from build123d import *

# Parameters (mm, degrees)
F0_W         = 26
F0_H         = 16
F0_W_2       = 20
F0_H_2       = 10
F1_DEPTH     = 20
F3_DEPTH     = 50
F4_SIZE      = 3
F5_T1_DEPTH  = 10
F5_T3_DEPTH  = 20
F5_T5_DEPTH  = 9.3860066631
F5_T7_DEPTH  = 9.3860066631
F5_T9_DEPTH  = 9.3860066631
F5_T11_DEPTH = 9.3860066631
F5_T13_DEPTH = 25.1433659759
F5_T15_DEPTH = 15.1433659759
F5_T21_DEPTH = 22.571682988
F5_T25_DEPTH = 12.571682988
F5_T32_DEPTH = 22.571682988
F5_T36_DEPTH = 12.571682988
F5_T43_DEPTH = 12.571682988
F5_T47_DEPTH = 22.571682988
F5_T54_DEPTH = 22.571682988
F5_T58_DEPTH = 12.571682988
F6_T1_DEPTH  = 9.3860066631
F6_T3_DEPTH  = 10
F6_T5_DEPTH  = 9.3860066631
F6_T7_DEPTH  = 25.1433659759
F6_T9_DEPTH  = 20
F6_T14_DEPTH = 9.3860066631
F6_T19_DEPTH = 9.3860066631
F6_T25_DEPTH = 22.571682988
F6_T30_DEPTH = 12.571682988
F6_T38_DEPTH = 22.571682988
F6_T43_DEPTH = 12.571682988
F6_T51_DEPTH = 22.571682988
F6_T56_DEPTH = 12.571682988
F6_T64_DEPTH = 12.571682988
F6_T69_DEPTH = 22.571682988
F7_SIZE      = 1


# Not quite as in the source:
# - a fillet or chamfer that OpenCascade refuses, or shapes differently, is made with other operations: its cross-section is extruded or revolved along the edge and cut away or added


with BuildPart() as f1:
    # F0 (on Front) → F1 (new body)
    with BuildSketch(Plane.XZ):
        with Locations((10, 5)):
            Rectangle(F0_W, F0_H)
        with Locations((10, 5)):
            Rectangle(F0_W_2, F0_H_2, mode=Mode.SUBTRACT)
    extrude(amount=F1_DEPTH)

    # F2 (on face) → F3 (join)
    with BuildSketch(Plane.YZ.offset(23)):
        Polygon((-18, 2.5), (-18, 5), (-18, 7.5), (-20, 7.5), (-20, 5), (-20, 2.5), align=None)
    extrude(amount=F3_DEPTH)

    # F4
    f4_edges = [f1.edges().sort_by_distance(p)[0] for p in [
        (-3, -10, 13),
        (23, -10, 13),
        (23, -18, 5),
        (-3, -10, -3),
        (23, -10, -3),
    ]]
    chamfer(f4_edges, length=F4_SIZE)

    # F5: chamfer of 1 on 12 edges, made by hand

    # F5_s2 → F5_t1 (cut)
    with BuildSketch(Plane.XY):
        Polygon((21, 0), (20, -1), (20, 0), align=None)
        Polygon((-1, 0), (0, -1), (0, 0), align=None)
    extrude(amount=F5_T1_DEPTH, mode=Mode.SUBTRACT)

    # F5_s4 → F5_t3 (cut)
    with BuildSketch(Plane.YZ):
        Polygon((0, 11), (-1, 10), (0, 10), align=None)
        Polygon((0, -1), (-1, 0), (0, 0), align=None)
    extrude(amount=F5_T3_DEPTH, mode=Mode.SUBTRACT)

    # F5_s6 → F5_t5 (cut)
    with BuildSketch(Plane(origin=(-3.3184544799, 0, 3.3184544799), x_dir=(0, 1, 0), z_dir=(0.7071067812, 0, -0.7071067812))):
        Polygon((0, -1.1213203436), (-1, -2.1213203436), (0, -2.1213203436), align=None)
    extrude(amount=F5_T5_DEPTH, mode=Mode.SUBTRACT)

    # F5_s8 → F5_t7 (cut)
    with BuildSketch(Plane(origin=(13.3184544799, 0, 13.3184544799), x_dir=(0, 1, 0), z_dir=(-0.7071067812, 0, -0.7071067812))):
        Polygon((0, 15.2634559673), (-1, 16.2634559673), (0, 16.2634559673), align=None)
    extrude(amount=F5_T7_DEPTH, mode=Mode.SUBTRACT)

    # F5_s10 → F5_t9 (cut)
    with BuildSketch(Plane(origin=(1.6815455201, 0, -1.6815455201), x_dir=(0, 1, 0), z_dir=(0.7071067812, 0, -0.7071067812))):
        Polygon((0, 22.3345237792), (-1, 23.3345237792), (0, 23.3345237792), align=None)
    extrude(amount=F5_T9_DEPTH, mode=Mode.SUBTRACT)

    # F5_s12 → F5_t11 (cut)
    with BuildSketch(Plane(origin=(8.3184544799, 0, 8.3184544799), x_dir=(0, 1, 0), z_dir=(-0.7071067812, 0, -0.7071067812))):
        Polygon((0, -8.1923881554), (-1, -9.1923881554), (0, -9.1923881554), align=None)
    extrude(amount=F5_T11_DEPTH, mode=Mode.SUBTRACT)

    # F5_s14 → F5_t13 (cut)
    with BuildSketch(Plane.YZ.offset(-2.571682988)):
        Polygon((0, -2), (-1, -3), (0, -3), align=None)
        Polygon((-1, 13), (0, 12), (0, 13), align=None)
    extrude(amount=F5_T13_DEPTH, mode=Mode.SUBTRACT)

    # F5_s16 → F5_t15 (cut)
    with BuildSketch(Plane.XY.offset(-2.571682988)):
        Polygon((22, 0), (23, -1), (23, 0), align=None)
        Polygon((-2, 0), (-3, -1), (-3, 0), align=None)
    extrude(amount=F5_T15_DEPTH, mode=Mode.SUBTRACT)


with BuildPart() as f5_tool19:
    # F5_s20 → F5_t21 (new body)
    with BuildSketch(Plane.YZ):
        Polygon((0, 11), (-1, 10), (0, 10), align=None)
    extrude(amount=F5_T21_DEPTH)

    split(bisect_by=Plane.YZ.offset(20), keep=Keep.TOP)


with BuildPart() as f5_tool23:
    # F5_s24 → F5_t25 (new body)
    with BuildSketch(Plane.XY.offset(12.571682988)):
        Polygon((21, 0), (20, -1), (20, 0), align=None)
    extrude(amount=-F5_T25_DEPTH)

    split(bisect_by=Plane.XY.offset(10), keep=Keep.TOP)


with BuildPart() as f5_tool19_1:
    add(f5_tool19.part)

    # F5_t27: intersect F5_tool23
    add(f5_tool23.part, mode=Mode.INTERSECT)


with BuildPart() as f1_1:
    add(f1.part)

    # F5_t17: cut F5_tool19
    add(f5_tool19_1.part, mode=Mode.SUBTRACT)


with BuildPart() as f5_tool30:
    # F5_s31 → F5_t32 (new body)
    with BuildSketch(Plane.YZ.offset(22.571682988)):
        Polygon((0, -1), (-1, 0), (0, 0), align=None)
    extrude(amount=-F5_T32_DEPTH)

    split(bisect_by=Plane.YZ.offset(20), keep=Keep.TOP)


with BuildPart() as f5_tool34:
    # F5_s35 → F5_t36 (new body)
    with BuildSketch(Plane.XY.offset(10)):
        Polygon((21, 0), (20, -1), (20, 0), align=None)
    extrude(amount=-F5_T36_DEPTH)

    split(bisect_by=Plane.XY, keep=Keep.BOTTOM)


with BuildPart() as f5_tool30_1:
    add(f5_tool30.part)

    # F5_t38: intersect F5_tool34
    add(f5_tool34.part, mode=Mode.INTERSECT)


with BuildPart() as f1_2:
    add(f1_1.part)

    # F5_t28: cut F5_tool30
    add(f5_tool30_1.part, mode=Mode.SUBTRACT)


with BuildPart() as f5_tool41:
    # F5_s42 → F5_t43 (new body)
    with BuildSketch(Plane.XY):
        Polygon((-1, 0), (0, -1), (0, 0), align=None)
    extrude(amount=F5_T43_DEPTH)

    split(bisect_by=Plane.XY.offset(10), keep=Keep.TOP)


with BuildPart() as f5_tool45:
    # F5_s46 → F5_t47 (new body)
    with BuildSketch(Plane.YZ.offset(-2.571682988)):
        Polygon((0, 11), (-1, 10), (0, 10), align=None)
    extrude(amount=F5_T47_DEPTH)

    split(bisect_by=Plane.YZ, keep=Keep.BOTTOM)


with BuildPart() as f5_tool41_1:
    add(f5_tool41.part)

    # F5_t49: intersect F5_tool45
    add(f5_tool45.part, mode=Mode.INTERSECT)


with BuildPart() as f1_3:
    add(f1_2.part)

    # F5_t39: cut F5_tool41
    add(f5_tool41_1.part, mode=Mode.SUBTRACT)


with BuildPart() as f5_tool52:
    # F5_s53 → F5_t54 (new body)
    with BuildSketch(Plane.YZ.offset(20)):
        Polygon((0, -1), (-1, 0), (0, 0), align=None)
    extrude(amount=-F5_T54_DEPTH)

    split(bisect_by=Plane.YZ, keep=Keep.BOTTOM)


with BuildPart() as f5_tool56:
    # F5_s57 → F5_t58 (new body)
    with BuildSketch(Plane.XY.offset(-2.571682988)):
        Polygon((-1, 0), (0, -1), (0, 0), align=None)
    extrude(amount=F5_T58_DEPTH)

    split(bisect_by=Plane.XY, keep=Keep.BOTTOM)


with BuildPart() as f5_tool52_1:
    add(f5_tool52.part)

    # F5_t60: intersect F5_tool56
    add(f5_tool56.part, mode=Mode.INTERSECT)


with BuildPart() as f1_4:
    add(f1_3.part)

    # F5_t50: cut F5_tool52
    add(f5_tool52_1.part, mode=Mode.SUBTRACT)

    # F6: chamfer of 1 on 10 edges, made by hand

    # F6_s2 → F6_t1 (cut)
    with BuildSketch(Plane(origin=(-3.3184544799, 0, 3.3184544799), x_dir=(0, 1, 0), z_dir=(0.7071067812, 0, -0.7071067812))):
        Polygon((-19, -2.1213203436), (-20, -1.1213203436), (-20, -2.1213203436), align=None)
    extrude(amount=F6_T1_DEPTH, mode=Mode.SUBTRACT)

    # F6_s4 → F6_t3 (cut)
    with BuildSketch(Plane.XY):
        Polygon((0, -19), (-1, -20), (0, -20), align=None)
        Polygon((20, -19), (21, -20), (20, -20), align=None)
    extrude(amount=F6_T3_DEPTH, mode=Mode.SUBTRACT)

    # F6_s6 → F6_t5 (cut)
    with BuildSketch(Plane(origin=(8.3184544799, 0, 8.3184544799), x_dir=(0, 1, 0), z_dir=(-0.7071067812, 0, -0.7071067812))):
        Polygon((-20, -8.1923881554), (-19, -9.1923881554), (-20, -9.1923881554), align=None)
    extrude(amount=F6_T5_DEPTH, mode=Mode.SUBTRACT)

    # F6_s8 → F6_t7 (cut)
    with BuildSketch(Plane.YZ.offset(-2.571682988)):
        Polygon((-19, -3), (-20, -2), (-20, -3), align=None)
        Polygon((-19, 13), (-20, 12), (-20, 13), align=None)
    extrude(amount=F6_T7_DEPTH, mode=Mode.SUBTRACT)

    # F6_s10 → F6_t9 (cut)
    with BuildSketch(Plane.YZ):
        Polygon((-19, 0), (-20, -1), (-20, 0), align=None)
        Polygon((-19, 10), (-20, 11), (-20, 10), align=None)
    extrude(amount=F6_T9_DEPTH, mode=Mode.SUBTRACT)


with BuildPart() as f6_tool12:
    # F6_s13 → F6_t14 (new body)
    with BuildSketch(Plane(origin=(1.6815455201, 0, -1.6815455201), x_dir=(0, 1, 0), z_dir=(0.7071067812, 0, -0.7071067812))):
        Polygon((-19, 23.3345237792), (-20, 22.3345237792), (-20, 23.3345237792), align=None)
    extrude(amount=F6_T14_DEPTH)

    split(bisect_by=Plane.XY.offset(7.5), keep=Keep.TOP)


with BuildPart() as f1_5:
    add(f1_4.part)

    # F6_t11: cut F6_tool12
    add(f6_tool12.part, mode=Mode.SUBTRACT)


with BuildPart() as f6_tool17:
    # F6_s18 → F6_t19 (new body)
    with BuildSketch(Plane(origin=(13.3184544799, 0, 13.3184544799), x_dir=(0, 1, 0), z_dir=(-0.7071067812, 0, -0.7071067812))):
        Polygon((-19, 16.2634559673), (-20, 15.2634559673), (-20, 16.2634559673), align=None)
    extrude(amount=F6_T19_DEPTH)

    split(bisect_by=Plane.XY.offset(2.5), keep=Keep.BOTTOM)


with BuildPart() as f1_6:
    add(f1_5.part)

    # F6_t16: cut F6_tool17
    add(f6_tool17.part, mode=Mode.SUBTRACT)


with BuildPart() as f6_tool23:
    # F6_s24 → F6_t25 (new body)
    with BuildSketch(Plane.YZ.offset(20)):
        Polygon((-19, 0), (-20, -1), (-20, 0), align=None)
    extrude(amount=-F6_T25_DEPTH)

    split(bisect_by=Plane(origin=(-1.5, 0, -1.5), x_dir=(0, 1, 0), z_dir=(0.7071067812, 0, 0.7071067812)), keep=Keep.TOP)

    split(bisect_by=Plane.YZ, keep=Keep.BOTTOM)


with BuildPart() as f6_tool28:
    # F6_s29 → F6_t30 (new body)
    with BuildSketch(Plane.XY.offset(-2.571682988)):
        Polygon((0, -19), (-1, -20), (0, -20), align=None)
    extrude(amount=F6_T30_DEPTH)

    split(bisect_by=Plane(origin=(-1.5, 0, -1.5), x_dir=(0, 1, 0), z_dir=(0.7071067812, 0, 0.7071067812)), keep=Keep.TOP)

    split(bisect_by=Plane.XY, keep=Keep.BOTTOM)


with BuildPart() as f6_tool23_1:
    add(f6_tool23.part)

    # F6_t33: intersect F6_tool28
    add(f6_tool28.part, mode=Mode.INTERSECT)


with BuildPart() as f1_7:
    add(f1_6.part)

    # F6_t21: cut F6_tool23
    add(f6_tool23_1.part, mode=Mode.SUBTRACT)


with BuildPart() as f6_tool36:
    # F6_s37 → F6_t38 (new body)
    with BuildSketch(Plane.YZ.offset(-2.571682988)):
        Polygon((-19, 10), (-20, 11), (-20, 10), align=None)
    extrude(amount=F6_T38_DEPTH)

    split(bisect_by=Plane.YZ, keep=Keep.BOTTOM)

    split(bisect_by=Plane(origin=(-6.5, 0, 6.5), x_dir=(0, 1, 0), z_dir=(0.7071067812, 0, -0.7071067812)), keep=Keep.TOP)


with BuildPart() as f6_tool41:
    # F6_s42 → F6_t43 (new body)
    with BuildSketch(Plane.XY):
        Polygon((0, -19), (-1, -20), (0, -20), align=None)
    extrude(amount=F6_T43_DEPTH)

    split(bisect_by=Plane.XY.offset(10), keep=Keep.TOP)

    split(bisect_by=Plane(origin=(-6.5, 0, 6.5), x_dir=(0, 1, 0), z_dir=(0.7071067812, 0, -0.7071067812)), keep=Keep.TOP)


with BuildPart() as f6_tool36_1:
    add(f6_tool36.part)

    # F6_t46: intersect F6_tool41
    add(f6_tool41.part, mode=Mode.INTERSECT)


with BuildPart() as f1_8:
    add(f1_7.part)

    # F6_t34: cut F6_tool36
    add(f6_tool36_1.part, mode=Mode.SUBTRACT)


with BuildPart() as f6_tool49:
    # F6_s50 → F6_t51 (new body)
    with BuildSketch(Plane.YZ.offset(22.571682988)):
        Polygon((-19, 0), (-20, -1), (-20, 0), align=None)
    extrude(amount=-F6_T51_DEPTH)

    split(bisect_by=Plane(origin=(11.5, 0, -11.5), x_dir=(0, 1, 0), z_dir=(-0.7071067812, 0, 0.7071067812)), keep=Keep.TOP)

    split(bisect_by=Plane.YZ.offset(20), keep=Keep.TOP)


with BuildPart() as f6_tool54:
    # F6_s55 → F6_t56 (new body)
    with BuildSketch(Plane.XY.offset(10)):
        Polygon((20, -19), (21, -20), (20, -20), align=None)
    extrude(amount=-F6_T56_DEPTH)

    split(bisect_by=Plane(origin=(11.5, 0, -11.5), x_dir=(0, 1, 0), z_dir=(-0.7071067812, 0, 0.7071067812)), keep=Keep.TOP)

    split(bisect_by=Plane.XY, keep=Keep.BOTTOM)


with BuildPart() as f6_tool49_1:
    add(f6_tool49.part)

    # F6_t59: intersect F6_tool54
    add(f6_tool54.part, mode=Mode.INTERSECT)


with BuildPart() as f1_9:
    add(f1_8.part)

    # F6_t47: cut F6_tool49
    add(f6_tool49_1.part, mode=Mode.SUBTRACT)


with BuildPart() as f6_tool62:
    # F6_s63 → F6_t64 (new body)
    with BuildSketch(Plane.XY.offset(12.571682988)):
        Polygon((20, -19), (21, -20), (20, -20), align=None)
    extrude(amount=-F6_T64_DEPTH)

    split(bisect_by=Plane(origin=(16.5, 0, 16.5), x_dir=(0, 1, 0), z_dir=(-0.7071067812, 0, -0.7071067812)), keep=Keep.TOP)

    split(bisect_by=Plane.XY.offset(10), keep=Keep.TOP)


with BuildPart() as f6_tool67:
    # F6_s68 → F6_t69 (new body)
    with BuildSketch(Plane.YZ):
        Polygon((-19, 10), (-20, 11), (-20, 10), align=None)
    extrude(amount=F6_T69_DEPTH)

    split(bisect_by=Plane(origin=(16.5, 0, 16.5), x_dir=(0, 1, 0), z_dir=(-0.7071067812, 0, -0.7071067812)), keep=Keep.TOP)

    split(bisect_by=Plane.YZ.offset(20), keep=Keep.TOP)


with BuildPart() as f6_tool62_1:
    add(f6_tool62.part)

    # F6_t72: intersect F6_tool67
    add(f6_tool67.part, mode=Mode.INTERSECT)


with BuildPart() as f1_10:
    add(f1_9.part)

    # F6_t60: cut F6_tool62
    add(f6_tool62_1.part, mode=Mode.SUBTRACT)

    # F7
    f7_edges = [f1_10.edges().sort_by_distance(p)[0] for p in [
        (-3, -20, 5),
    ]]
    chamfer(f7_edges, length=F7_SIZE)


solid = f1_10.part
Part model, mm, in its own coordinate system. A direction names the side the tool comes from. Give positions to 0.01 mm unless a question says otherwise; leave off trailing zeros. Order: outer loops, then holes, each group sorted by start corner. A loop starts at its lowest first (then second) coordinate and runs counter-clockwise, first axis right, second up. Notation, with made-up numbers: (25, 85.5) -> (35, 85.5) arc R22 cw to (35, 105.5) -> close; hole circle Ø6 at (56, -34.75). An arc over 180 degrees is marked (long way). Use one line per item in the form item = value.
(1) Saw through at D-D (x = 56). Write the cut outline in (y, z).
Solution:
outline = (-20, 2.5) -> (-18, 2.5) -> (-18, 7.5) -> (-20, 7.5) -> close
(2) Pull direction Z, two halves, no side cores. Call faces 6 (the face through (10, -10, -3)), 7 (the face through (-1.12, -19.51, 11.16)), 8 (the face through (10, -10, 10)): +Z half, -Z half, draft (parallel to the pull), parting line (faces both ways), or undercut.
Solution:
face_6 = -Z half
face_7 = +Z half
face_8 = undercut
(3) Saw through at B-B (x = 5). Write the cut outline in (y, z), then the cut area to 3 significant figures.
Solution:
outline = (-20, -2) -> (-19, -3) -> (-1, -3) -> (0, -2) -> (0, -1) -> (-1, 0) -> (-19, 0) -> (-20, -1) -> close; (-20, 11) -> (-19, 10) -> (-1, 10) -> (0, 11) -> (0, 12) -> (-1, 13) -> (-19, 13) -> (-20, 12) -> close
area = 116 mm²
(4) Saw through at A-A (y = -17). Write the cut outline in (x, z).
Solution:
outline = (-3, 0) -> (0, -3) -> (20, -3) -> (23, 0) -> (23, 2.5) -> (25, 2.5) -> (25, 7.5) -> (23, 7.5) -> (23, 10) -> (20, 13) -> (0, 13) -> (-3, 10) -> close; hole (0, 0) -> (20, 0) -> (20, 10) -> (0, 10) -> close
(5) Tool access for faces 1 (the face through (21.16, -0.49, -1.12)), 2 (the face through (49, -18, 5)), 3 (the face through (0, -10, 5)), 4 (the face through (48, -19, 7.5)), 5 (the face through (48, -19, 2.5)): list every direction of +Z, -Z, +X, -X, +Y, -Y with a clear straight run to the whole face (end or side of a thin tool).
Solution:
face_1 = -Z, +X, +Y
face_2 = +Z, -Z, +X, +Y
face_3 = +Y, -Y
face_4 = +Z, +X, +Y, -Y
face_5 = -Z, +X, +Y, -Y
(6) Drill centre lines: line 1 (X direction, y = -5.75, z = 2); line 2 (Z direction, x = 5, y = -7); line 3 (Z direction, x = 21, y = -8.75). Where is each one in solid material? Low to high. Write a range as from..to.
Solution:
line_1 = -3..0, 20..23
line_2 = -3..0, 10..13
line_3 = -2..12
(7) Flat gauge pins, fed straight in: P1, Ø5.5, axis at x = 59.5, z = 5, coming from the +Y side; P2, Ø5, axis at x = 24.5, z = 0, coming from the +Y side; P3, Ø5, axis at y = -13, z = 3, coming from the +X side; P4, Ø1.5, axis at x = 50.5, y = -16.5, coming from the -Z side. Where does each tip first touch, or does it go through?
Solution:
P1 = -18
P2 = -0.03
P3 = 23.5
P4 = through
(8) Saw through at C-C (z = 3.75). Write the cut outline in (x, y).
Solution:
outline = (-3, -19) -> (-2, -20) -> (-1, -20) -> (0, -19) -> (0, -1) -> (-1, 0) -> (-2, 0) -> (-3, -1) -> close; (20, -19) -> (21, -20) -> (73, -20) -> (73, -18) -> (26, -18) -> (23, -15) -> (23, -1) -> (22, 0) -> (21, 0) -> (20, -1) -> close
